Answer from the drawing. Dimensions are ordinates in mm from the lowest x, y and z of the part. A direction names the side the tool comes from. Round coordinates to 2 decimals unless told otherwise and drop trailing zeros. Loops run counter-clockwise (first coordinate to the right, second up) from the corner with the lowest first, then second, coordinate; pieces in that order, holes last. Notation, with made-up numbers: M 45.5,72.5 L 91.5,72.5 A25 ccw 91.5,88.5 Z; hole C 32.25,64 d3. An arc over 180 degrees is marked long. Answer as CSV lines item,"result".
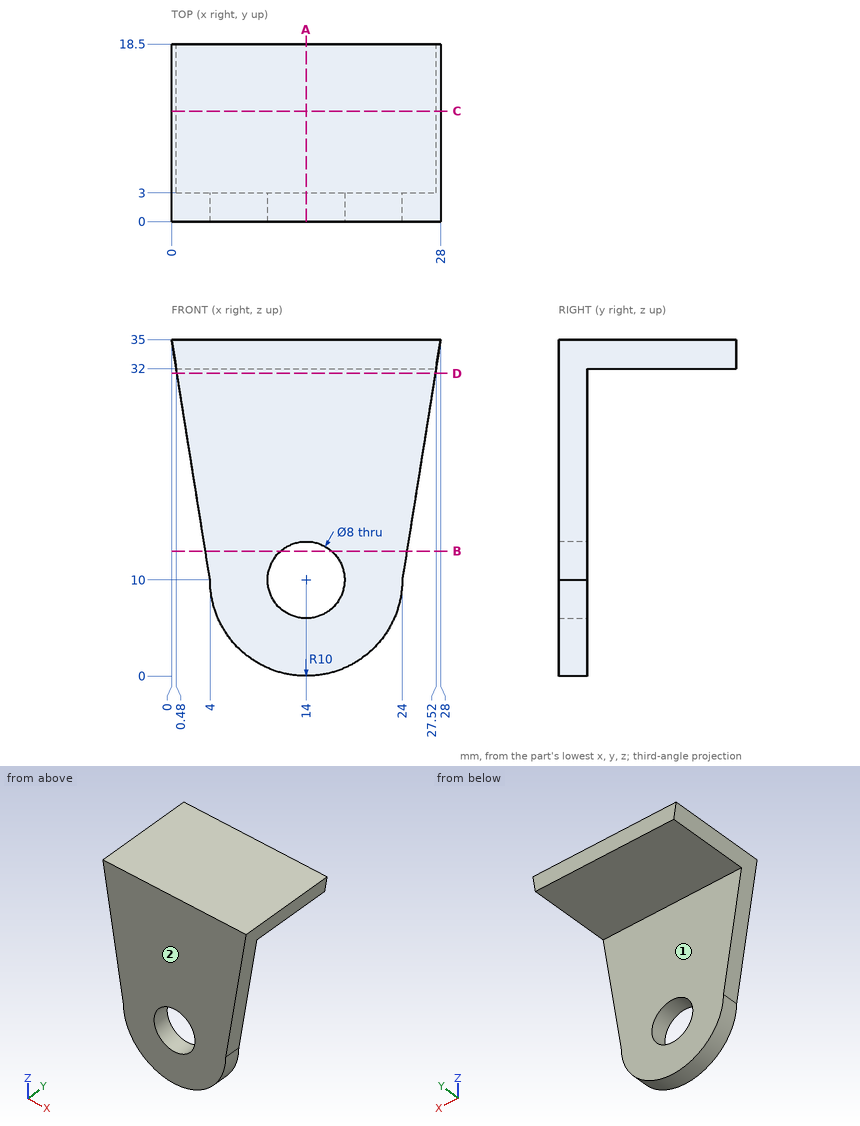
1) Find section C-C, the plane y = 11.5. Give the vertices of the cut face in (x, z), then the cut area to 3 significant figures.
Evaluation:
outline,"M 0,35 L 0.48,32 L 27.52,32 L 28,35 Z"
area,"82.6 mm^2"
2) Straight lines are drawn through the part: line 1 (Z direction, x = 14, y = 1.7); line 2 (X direction, y = 1.45, z = 10); line 3 (Z direction, x = 2.25, y = 7). For each, find the intervals that lie inside material, in ascending order.
Evaluation:
line 1,"z = 0 to 6, 14 to 35"
line 2,"x = 4 to 10, 18 to 24"
line 3,"z = 32 to 35"
3) A tool of negligible diameter and unlimited length cuts with its end or side. For the marked faces 1 and 2, from which of +Z, -Z, +X, -X, +Y, -Y can it reach the whole face along a straight path? Write none if from no direction.
Evaluation:
face 1,"-Z, +X, -X, +Y"
face 2,"+Z, -Z, +X, -X, -Y"
4) Find section B-B, the plane z = 13. Give the vertices of the cut face in (x, y), then the cut area to 3 significant figures.
Evaluation:
outline,"M 3.52,0 L 11.35,0 L 11.35,3 L 3.52,3 Z; M 16.65,0 L 24.48,0 L 24.48,3 L 16.65,3 Z"
area,"47.0 mm^2"
5) Each of these flat-tipped pins is pushed along its axis until it touches: P1, Ø5, axis at x = 10, z = 22, coming from the +Y side; P2, Ø1.5, axis at x = 7.5, y = 10.5, coming from the -Z side; P3, Ø2, axis at y = 5, z = 15, coming from the +X side. Where does it stop, or does it pass through?
Evaluation:
P1,"stops at y = 3"
P2,"stops at z = 32"
P3,"passes through"
6) Find section D-D, the plane z = 31.5. Give the vertices of the cut face in (x, y).
Evaluation:
outline,"M 0.56,0 L 27.44,0 L 27.44,3 L 0.56,3 Z"
7) Find section A-A, the plane x = 14. Give the vertices of the cut face in (y, z).
Evaluation:
outline,"M 0,0 L 3,0 L 3,6 L 0,6 Z; M 0,14 L 3,14 L 3,32 L 18.5,32 L 18.5,35 L 0,35 Z"
